Design review of the part built by this model. Coordinates are the model's own, in mm. A direction names the side the tool comes from. Coordinates: 2 decimals unless noted, no trailing zeros. Loops run counter-clockwise (first coordinate to the right, second up) from the corner with the lowest first, then second, coordinate; pieces in that order, holes last. Notation, with made-up numbers: M -27.75,23.25 L 14.25,23.25 A10 ccw 14.25,41.25 Z; hole C 31.5,-19 d9. An arc over 180 degrees is marked long. One line per item, written item: value.
```python
from build123d import *

# Parameters (mm, degrees)
F0_W         = 38.1
F0_H         = 101.6
F1_DEPTH     = 15.875
F2_W         = 27.94
F2_H         = 76.5175
F3_DEPTH     = 12.7
F4_W         = 29.8249544576
F4_H         = 10.7437949628
F5_DEPTH     = 100.23084
F6_T4_DEPTH  = 100.23084
F6_T10_DEPTH = 100.23084
F6_T16_DEPTH = 100.23084
F6_T23_DEPTH = 100.23084
F6_T29_DEPTH = 100.23084
F6_T35_DEPTH = 100.23084
F6_T41_DEPTH = 100.23084
F6_T47_DEPTH = 100.23084
F6_T54_DEPTH = 100.23084
F6_T60_DEPTH = 100.23084
F6_T63_DEPTH = 127


# Not quite as in the source:
# - a fillet or chamfer that OpenCascade refuses, or shapes differently, is made with other operations: its cross-section is extruded or revolved along the edge and cut away or added


with BuildPart() as f1:
    # F0 (on Front) → F1 (new body)
    with BuildSketch(Plane.XZ):
        with Locations((-29.7519958138, -32.7344046354)):
            Rectangle(F0_W, F0_H)
    extrude(amount=F1_DEPTH)

    # F2 (on face) → F3 (cut)
    with BuildSketch(Plane.XZ.offset(15.875)):
        with Locations((-29.7519958138, -27.8131546354)):
            Rectangle(F2_W, F2_H)
    extrude(amount=-F3_DEPTH, mode=Mode.SUBTRACT)

    # F4 (on face) → F5 (cut)
    with BuildSketch(Plane.XY.offset(18.0655953646)):
        with Locations((-29.750072863, -8.0031603575)):
            Rectangle(F4_W, F4_H)
    extrude(amount=-F5_DEPTH, mode=Mode.SUBTRACT)

    # F6: fillet of radius 5.08 on 4 edges, made by hand


with BuildPart() as f6_tool2:
    # F6_s3 → F6_t4 (new body)
    with BuildSketch(Plane.XY.offset(18.0655953646)):
        with BuildLine():
            ThreePointArc((-19.9175956342, -13.3750578389), (-16.3254931857, -11.8871602873), (-14.8375956342, -8.2950578389))
            Line((-14.8375956342, -8.2950578389), (-14.8375956342, -13.3750578389))
            Line((-14.8375956342, -13.3750578389), (-19.9175956342, -13.3750578389))
        make_face()
    extrude(amount=-F6_T4_DEPTH)

    split(bisect_by=Plane.YZ.offset(-15.7819958138), keep=Keep.BOTTOM)

    split(bisect_by=Plane.XY.offset(10.4455953646), keep=Keep.TOP)


with BuildPart() as f1_1:
    add(f1.part)

    # F6_t1: union F6_tool2
    add(f6_tool2.part)


with BuildPart() as f6_tool8:
    # F6_s9 → F6_t10 (new body)
    with BuildSketch(Plane.XY.offset(18.0655953646)):
        with BuildLine():
            ThreePointArc((-19.9175956342, -13.3750578389), (-16.3254931857, -11.8871602873), (-14.8375956342, -8.2950578389))
            Line((-14.8375956342, -8.2950578389), (-14.8375956342, -13.3750578389))
            Line((-14.8375956342, -13.3750578389), (-19.9175956342, -13.3750578389))
        make_face()
    extrude(amount=-F6_T10_DEPTH)

    split(bisect_by=Plane.YZ.offset(-15.7819958138), keep=Keep.TOP)

    split(bisect_by=Plane.XY.offset(10.4455953646), keep=Keep.TOP)


with BuildPart() as f1_2:
    add(f1_1.part)

    # F6_t7: union F6_tool8
    add(f6_tool8.part)


with BuildPart() as f6_tool14:
    # F6_s15 → F6_t16 (new body)
    with BuildSketch(Plane.XY.offset(18.0655953646)):
        with BuildLine():
            ThreePointArc((-19.9175956342, -13.3750578389), (-16.3254931857, -11.8871602873), (-14.8375956342, -8.2950578389))
            Line((-14.8375956342, -8.2950578389), (-14.8375956342, -13.3750578389))
            Line((-14.8375956342, -13.3750578389), (-19.9175956342, -13.3750578389))
        make_face()
    extrude(amount=-F6_T16_DEPTH)

    split(bisect_by=Plane.XY.offset(-66.0719046354), keep=Keep.TOP)

    split(bisect_by=Plane.YZ.offset(-15.7819958138), keep=Keep.TOP)

    split(bisect_by=Plane.XY.offset(10.4455953646), keep=Keep.BOTTOM)


with BuildPart() as f1_3:
    add(f1_2.part)

    # F6_t13: union F6_tool14
    add(f6_tool14.part)


with BuildPart() as f6_tool21:
    # F6_s22 → F6_t23 (new body)
    with BuildSketch(Plane.XY.offset(18.0655953646)):
        with BuildLine():
            ThreePointArc((-19.9175956342, -13.3750578389), (-16.3254931857, -11.8871602873), (-14.8375956342, -8.2950578389))
            Line((-14.8375956342, -8.2950578389), (-14.8375956342, -13.3750578389))
            Line((-14.8375956342, -13.3750578389), (-19.9175956342, -13.3750578389))
        make_face()
    extrude(amount=-F6_T23_DEPTH)

    split(bisect_by=Plane.XY.offset(-66.0719046354), keep=Keep.BOTTOM)

    split(bisect_by=Plane.YZ.offset(-15.7819958138), keep=Keep.BOTTOM)


with BuildPart() as f1_4:
    add(f1_3.part)

    # F6_t20: union F6_tool21
    add(f6_tool21.part)


with BuildPart() as f6_tool27:
    # F6_s28 → F6_t29 (new body)
    with BuildSketch(Plane.XY.offset(18.0655953646)):
        with BuildLine():
            ThreePointArc((-19.9175956342, -13.3750578389), (-16.3254931857, -11.8871602873), (-14.8375956342, -8.2950578389))
            Line((-14.8375956342, -8.2950578389), (-14.8375956342, -13.3750578389))
            Line((-14.8375956342, -13.3750578389), (-19.9175956342, -13.3750578389))
        make_face()
    extrude(amount=-F6_T29_DEPTH)

    split(bisect_by=Plane.XY.offset(-66.0719046354), keep=Keep.BOTTOM)

    split(bisect_by=Plane.YZ.offset(-15.7819958138), keep=Keep.TOP)


with BuildPart() as f1_5:
    add(f1_4.part)

    # F6_t26: union F6_tool27
    add(f6_tool27.part)


with BuildPart() as f6_tool33:
    # F6_s34 → F6_t35 (new body)
    with BuildSketch(Plane.XY.offset(18.0655953646)):
        with BuildLine():
            ThreePointArc((-39.5825500917, -13.3750578389), (-43.1746525402, -11.8871602873), (-44.6625500917, -8.2950578389))
            Line((-44.6625500917, -8.2950578389), (-44.6625500917, -13.3750578389))
            Line((-44.6625500917, -13.3750578389), (-39.5825500917, -13.3750578389))
        make_face()
    extrude(amount=-F6_T35_DEPTH)

    split(bisect_by=Plane.YZ.offset(-43.7219958138), keep=Keep.TOP)

    split(bisect_by=Plane.XY.offset(10.4455953646), keep=Keep.TOP)


with BuildPart() as f1_6:
    add(f1_5.part)

    # F6_t32: union F6_tool33
    add(f6_tool33.part)


with BuildPart() as f6_tool39:
    # F6_s40 → F6_t41 (new body)
    with BuildSketch(Plane.XY.offset(18.0655953646)):
        with BuildLine():
            ThreePointArc((-39.5825500917, -13.3750578389), (-43.1746525402, -11.8871602873), (-44.6625500917, -8.2950578389))
            Line((-44.6625500917, -8.2950578389), (-44.6625500917, -13.3750578389))
            Line((-44.6625500917, -13.3750578389), (-39.5825500917, -13.3750578389))
        make_face()
    extrude(amount=-F6_T41_DEPTH)

    split(bisect_by=Plane.YZ.offset(-43.7219958138), keep=Keep.BOTTOM)

    split(bisect_by=Plane.XY.offset(10.4455953646), keep=Keep.TOP)


with BuildPart() as f1_7:
    add(f1_6.part)

    # F6_t38: union F6_tool39
    add(f6_tool39.part)


with BuildPart() as f6_tool45:
    # F6_s46 → F6_t47 (new body)
    with BuildSketch(Plane.XY.offset(18.0655953646)):
        with BuildLine():
            ThreePointArc((-39.5825500917, -13.3750578389), (-43.1746525402, -11.8871602873), (-44.6625500917, -8.2950578389))
            Line((-44.6625500917, -8.2950578389), (-44.6625500917, -13.3750578389))
            Line((-44.6625500917, -13.3750578389), (-39.5825500917, -13.3750578389))
        make_face()
    extrude(amount=-F6_T47_DEPTH)

    split(bisect_by=Plane.YZ.offset(-43.7219958138), keep=Keep.BOTTOM)

    split(bisect_by=Plane.XY.offset(-66.0719046354), keep=Keep.TOP)

    split(bisect_by=Plane.XY.offset(10.4455953646), keep=Keep.BOTTOM)


with BuildPart() as f1_8:
    add(f1_7.part)

    # F6_t44: union F6_tool45
    add(f6_tool45.part)


with BuildPart() as f6_tool52:
    # F6_s53 → F6_t54 (new body)
    with BuildSketch(Plane.XY.offset(18.0655953646)):
        with BuildLine():
            ThreePointArc((-39.5825500917, -13.3750578389), (-43.1746525402, -11.8871602873), (-44.6625500917, -8.2950578389))
            Line((-44.6625500917, -8.2950578389), (-44.6625500917, -13.3750578389))
            Line((-44.6625500917, -13.3750578389), (-39.5825500917, -13.3750578389))
        make_face()
    extrude(amount=-F6_T54_DEPTH)

    split(bisect_by=Plane.YZ.offset(-43.7219958138), keep=Keep.TOP)

    split(bisect_by=Plane.XY.offset(-66.0719046354), keep=Keep.BOTTOM)


with BuildPart() as f1_9:
    add(f1_8.part)

    # F6_t51: union F6_tool52
    add(f6_tool52.part)


with BuildPart() as f6_tool58:
    # F6_s59 → F6_t60 (new body)
    with BuildSketch(Plane.XY.offset(18.0655953646)):
        with BuildLine():
            ThreePointArc((-39.5825500917, -13.3750578389), (-43.1746525402, -11.8871602873), (-44.6625500917, -8.2950578389))
            Line((-44.6625500917, -8.2950578389), (-44.6625500917, -13.3750578389))
            Line((-44.6625500917, -13.3750578389), (-39.5825500917, -13.3750578389))
        make_face()
    extrude(amount=-F6_T60_DEPTH)

    split(bisect_by=Plane.YZ.offset(-43.7219958138), keep=Keep.BOTTOM)

    split(bisect_by=Plane.XY.offset(-66.0719046354), keep=Keep.BOTTOM)


with BuildPart() as f1_10:
    add(f1_9.part)

    # F6_t57: union F6_tool58
    add(f6_tool58.part)

    # F6_s64 → F6_t63 (cut)
    with BuildSketch(Plane.XY.offset(-96.2344046354)):
        with BuildLine():
            ThreePointArc((-10.7019958138, -10.795), (-12.1898933654, -14.3871024484), (-15.7819958138, -15.875))
            Line((-15.7819958138, -15.875), (-10.7019958138, -15.875))
            Line((-10.7019958138, -15.875), (-10.7019958138, -10.795))
        make_face()
        with BuildLine():
            ThreePointArc((-43.7219958138, -15.875), (-47.3140982623, -14.3871024484), (-48.8019958138, -10.795))
            Line((-48.8019958138, -10.795), (-48.8019958138, -15.875))
            Line((-48.8019958138, -15.875), (-43.7219958138, -15.875))
        make_face()
    extrude(amount=F6_T63_DEPTH, mode=Mode.SUBTRACT)


solid = f1_10.part
```
(1) Tool access review of faces 1 (the flat face through (-30, -8, -82.165)), 2 (the cylindrical face through (-12.151, -14.347, -33.446)), 3 (the flat face through (-30, -15, 10.446)): name each direction out of +Z, -Z, +X, -X, +Y, -Y from which nothing blocks a thin tool from reaching the whole face with its end or side.
Reply:
face 1: +Z
face 2: +Z, -Z, +X, -Y
face 3: -Y
(2) To check wall thickness, follow line 1 along Z through (x, y) = (-35.5, -15); line 2 along X through (y, z) = (-6, -64); line 3 along Y through (x, z) = (-25, -76.5) (3 decimals). State the ranges of each line that lie inside material, in increasing order. Write a range as [from, to].
Reply:
line 1: z = [-83.53, -66.07], [10.45, 18.07]
line 2: x = [-48.8, -44.66], [-14.84, -10.7]
line 3: y = [-15.875, -13.375], [-2.631, 0]
(3) We need section A-A on z = -75. State the section outline as (x, y) points (3 decimals).
Reply:
outline: M -48.802,-10.795 A5.08 ccw -43.722,-15.875 L -15.782,-15.875 A5.08 ccw -10.702,-10.795 L -10.702,0 L -48.802,0 Z; hole M -44.663,-8.295 A5.08 ccw -39.583,-13.375 L -19.918,-13.375 A5.08 ccw -14.838,-8.295 L -14.838,-2.631 L -44.663,-2.631 Z
(4) We need section D-D on z = -56.5. State the section outline as (x, y) points (3 decimals).
Reply:
outline: M -48.802,-10.795 A5.08 ccw -43.722,-15.875 L -43.722,-11.24 A5.08 cw -44.663,-8.295 L -44.663,-2.631 L -14.838,-2.631 L -14.838,-8.295 A5.08 cw -15.782,-11.245 L -15.782,-15.875 A5.08 ccw -10.702,-10.795 L -10.702,0 L -48.802,0 Z
(5) Mouldability with a two-part tool opening along Y and no side actions: class faces 4 (the flat face through (-30, -15.875, -75)), 5 (the flat face through (-30, -15, -66.072)), 6 (the flat face through (-30, 0, -32)), 7 (the cylindrical face through (-44.163, -10.492, -31.348)) as released by +Y, released by -Y, zero draft, split by the parting line, or undercut.
Reply:
face 4: released by -Y
face 5: zero draft
face 6: released by +Y
face 7: undercut
(6) Insertion check: pin 1 (1.4 mm diameter, centred on y = -14, z = -20, fed in from -X); pin 2 (3 mm diameter, centred on x = -32, y = -9, fed in from +Z); pin 3 (5 mm diameter, centred on y = -14, z = -41.5, fed in from +X). Each pin has a flat end and moves straight along its axis. Give the tip position at first contact, or say it passes through.
Reply:
pin 1: stops at x = -48.14
pin 2: stops at z = -82.17
pin 3: stops at x = -10.75
(7) We need section B-B on x = -38. State the section outline as (y, z) points (3 decimals), then the cut area to 3 significant figures.
Reply:
outline: M -15.875,-83.534 L 0,-83.534 L 0,18.066 L -2.631,18.066 L -2.631,-82.165 L -13.375,-82.165 L -13.375,-66.072 L -15.875,-66.072 Z; M -15.875,10.446 L -13.375,10.446 L -13.375,18.066 L -15.875,18.066 Z
area: 345 mm2
(8) We need section C-C on y = -4.25. State the section outline as (x, z) points.
Reply:
outline: M -48.8,-83.53 L -10.7,-83.53 L -10.7,18.07 L -14.84,18.07 L -14.84,-82.17 L -44.66,-82.17 L -44.66,18.07 L -48.8,18.07 Z
